from build123d import *

# Parameters (mm, degrees)
BOSS_EXTRUDE1_DEPTH     = 40
SKETCH2_W               = 10
SKETCH2_H               = 10
BOSS_EXTRUDE2_DEPTH     = 80
SKETCH3_R               = 1.5
CUT_EXTRUDE1_DEPTH      = 48.749345545
SKETCH4_R               = 1.5
BOSS_EXTRUDE3_DEPTH     = 10
CHAMFER1_SIZE           = 23.551326066
CHAMFER1_SIZE_2         = 12
CHAMFER2_SIZE           = 4
CHAMFER3_SIZE           = 4
CHAMFER4_SIZE           = 12
SKETCH7_R               = 1.5
CUT_EXTRUDE3_DEPTH      = 104.330973091
CUT_EXTRUDE2_DEPTH      = 103.553839519
CUT_EXTRUDE2_DEPTH_BACK = 2
CHAMFER5_SIZE           = 7
SKETCH8_R               = 5.15
CUT_EXTRUDE4_DEPTH      = 5.5
SKETCH9_R               = 2.75
CUT_EXTRUDE5_DEPTH      = 95.417371283
CHAMFER6_SIZE           = 2.5


# Some blends are built 0.0001 mm under size
with BuildPart() as part:
    # Sketch1 → Boss-Extrude1 (new, symmetric)
    with BuildSketch(Plane(origin=(0, 0, 0), x_dir=(0, 0, -1), z_dir=(1, 0, 0))):
        Polygon((0, 4), (0, 15), (-4, 15), (-4, -15), (0, -15), (0, -4), (1, -4), (1, 4), align=None)
    extrude(amount=BOSS_EXTRUDE1_DEPTH, both=True)

    # Sketch2 → Boss-Extrude2 (add)
    with BuildSketch(Plane.ZY.offset(40)):
        with Locations((9, -2)):
            Rectangle(SKETCH2_W, SKETCH2_H)
    extrude(amount=-BOSS_EXTRUDE2_DEPTH)

    # Sketch3 → Cut-Extrude1 (cut, through all)
    with BuildSketch(Plane.XZ.offset(7)):
        with Locations(Location((-28.7, 7.55, 0), (0, 0, 270))):
            Circle(SKETCH3_R)
        with Locations(Location((28.7, 7.55, 0), (0, 0, 270))):
            Circle(SKETCH3_R)
    extrude(amount=-CUT_EXTRUDE1_DEPTH, mode=Mode.SUBTRACT)

    # Sketch4 → Boss-Extrude3 (add)
    with BuildSketch(Plane.XZ.offset(7)):
        Polygon((-40, 14), (-29.75, 14), (-29.75, 72.7), (-25.75, 72.7), (-25.75, 84.7), (25.75, 84.7), (25.75, 72.7), (29.75, 72.7), (29.75, 14), (40, 14), (40, 92.7), (-40, 92.7), align=None)
        with Locations(Location((-28.7, 77.65, 0), (0, 0, 270))):
            Circle(SKETCH4_R, mode=Mode.SUBTRACT)
        with Locations(Location((28.7, 77.65, 0), (0, 0, 90))):
            Circle(SKETCH4_R, mode=Mode.SUBTRACT)
    extrude(amount=-BOSS_EXTRUDE3_DEPTH)

    # Chamfer1
    # the kernel refuses this chamfer: 23.551326066, 12 mm, written as the material it adds along each edge
    with BuildSketch(Plane(origin=(-40, 3, 4), x_dir=(0, -0.017531984409911095, 0.9998463029499337), z_dir=(1, 0, 0))) as chamfer1_piece_1_section:
        Polygon((CHAMFER1_SIZE * 0.999846302953, -CHAMFER1_SIZE * 0.01753198441), (-CHAMFER1_SIZE_2 * 0.0175319844099, -CHAMFER1_SIZE_2 * 0.99984630295), (0, 0), align=None)
    chamfer1_piece_1 = extrude(amount=80, mode=Mode.PRIVATE)
    chamfer1_piece_1 = split(chamfer1_piece_1, bisect_by=Plane(origin=(-34.875, 4.887878827, 14), z_dir=(0, 0, 1)), keep=Keep.TOP, mode=Mode.PRIVATE)
    chamfer1_piece_1 = split(chamfer1_piece_1, bisect_by=Plane(origin=(-29.75, 4.887878827, 19.058840597), z_dir=(-1, 0, 0)), keep=Keep.TOP, mode=Mode.PRIVATE)
    add(chamfer1_piece_1)
    with BuildSketch(Plane(origin=(-40, 3, 4), x_dir=(0, -0.017531984409911095, 0.9998463029499337), z_dir=(1, 0, 0))) as chamfer1_piece_2_section:
        Polygon((CHAMFER1_SIZE * 0.999846302953, -CHAMFER1_SIZE * 0.01753198441), (-CHAMFER1_SIZE_2 * 0.0175319844099, -CHAMFER1_SIZE_2 * 0.99984630295), (0, 0), align=None)
    chamfer1_piece_2 = extrude(amount=80, mode=Mode.PRIVATE)
    chamfer1_piece_2 = split(chamfer1_piece_2, bisect_by=Plane(origin=(-34.907327213, 7.791187199, 14), z_dir=(0, 0, -1)), keep=Keep.TOP, mode=Mode.PRIVATE)
    chamfer1_piece_2 = split(chamfer1_piece_2, bisect_by=Plane(origin=(-29.75, 7.791187199, 8.24071688), z_dir=(-1, 0, 0)), keep=Keep.TOP, mode=Mode.PRIVATE)
    chamfer1_piece_2 = chamfer1_piece_2 - Plane(origin=(-28.7, 7.791187199, 7.55), x_dir=(0, 0, -1), z_dir=(0, -1, 0)) * Cylinder(1.5, 255, mode=Mode.PRIVATE)
    chamfer1_piece_2 = split(chamfer1_piece_2, bisect_by=Plane(origin=(-34.907327213, 15, 8.24071688), z_dir=(0, -1, 0)), keep=Keep.TOP, mode=Mode.PRIVATE)
    add(chamfer1_piece_2)
    with BuildSketch(Plane(origin=(-40, 3, 4), x_dir=(0, -0.017531984409911095, 0.9998463029499337), z_dir=(1, 0, 0))) as chamfer1_piece_3_section:
        Polygon((CHAMFER1_SIZE * 0.999846302953, -CHAMFER1_SIZE * 0.01753198441), (-CHAMFER1_SIZE_2 * 0.0175319844099, -CHAMFER1_SIZE_2 * 0.99984630295), (0, 0), align=None)
    chamfer1_piece_3 = extrude(amount=80, mode=Mode.PRIVATE)
    chamfer1_piece_3 = split(chamfer1_piece_3, bisect_by=Plane(origin=(3.218e-06, 7.789653484, 14), z_dir=(0, 0, -1)), keep=Keep.TOP, mode=Mode.PRIVATE)
    chamfer1_piece_3 = split(chamfer1_piece_3, bisect_by=Plane(origin=(-29.75, 7.789653484, 8.251914963), z_dir=(1, 0, 0)), keep=Keep.TOP, mode=Mode.PRIVATE)
    chamfer1_piece_3 = split(chamfer1_piece_3, bisect_by=Plane(origin=(29.75, 7.789653484, 8.251914963), z_dir=(-1, 0, 0)), keep=Keep.TOP, mode=Mode.PRIVATE)
    chamfer1_piece_3 = chamfer1_piece_3 - Plane(origin=(28.7, 7.789653484, 7.55), x_dir=(0, 0, -1), z_dir=(0, -1, 0)) * Cylinder(1.5, 255, mode=Mode.PRIVATE)
    chamfer1_piece_3 = chamfer1_piece_3 - Plane(origin=(-28.7, 7.789653484, 7.55), x_dir=(0, 0, -1), z_dir=(0, -1, 0)) * Cylinder(1.5, 255, mode=Mode.PRIVATE)
    chamfer1_piece_3 = split(chamfer1_piece_3, bisect_by=Plane(origin=(3.218e-06, 15, 8.251914963), z_dir=(0, -1, 0)), keep=Keep.TOP, mode=Mode.PRIVATE)
    add(chamfer1_piece_3)
    with BuildSketch(Plane(origin=(-40, 3, 4), x_dir=(0, -0.017531984409911095, 0.9998463029499337), z_dir=(1, 0, 0))) as chamfer1_piece_4_section:
        Polygon((CHAMFER1_SIZE * 0.999846302953, -CHAMFER1_SIZE * 0.01753198441), (-CHAMFER1_SIZE_2 * 0.0175319844099, -CHAMFER1_SIZE_2 * 0.99984630295), (0, 0), align=None)
    chamfer1_piece_4 = extrude(amount=80, mode=Mode.PRIVATE)
    chamfer1_piece_4 = split(chamfer1_piece_4, bisect_by=Plane(origin=(34.875, 4.887878827, 14), z_dir=(0, 0, 1)), keep=Keep.TOP, mode=Mode.PRIVATE)
    chamfer1_piece_4 = split(chamfer1_piece_4, bisect_by=Plane(origin=(29.75, 4.887878827, 19.058840597), z_dir=(1, 0, 0)), keep=Keep.TOP, mode=Mode.PRIVATE)
    add(chamfer1_piece_4)
    with BuildSketch(Plane(origin=(-40, 3, 4), x_dir=(0, -0.017531984409911095, 0.9998463029499337), z_dir=(1, 0, 0))) as chamfer1_piece_5_section:
        Polygon((CHAMFER1_SIZE * 0.999846302953, -CHAMFER1_SIZE * 0.01753198441), (-CHAMFER1_SIZE_2 * 0.0175319844099, -CHAMFER1_SIZE_2 * 0.99984630295), (0, 0), align=None)
    chamfer1_piece_5 = extrude(amount=80, mode=Mode.PRIVATE)
    chamfer1_piece_5 = split(chamfer1_piece_5, bisect_by=Plane(origin=(34.907327332, 7.791187313, 14), z_dir=(0, 0, -1)), keep=Keep.TOP, mode=Mode.PRIVATE)
    chamfer1_piece_5 = split(chamfer1_piece_5, bisect_by=Plane(origin=(29.75, 7.791187313, 8.240716948), z_dir=(1, 0, 0)), keep=Keep.TOP, mode=Mode.PRIVATE)
    chamfer1_piece_5 = chamfer1_piece_5 - Plane(origin=(28.7, 7.791187313, 7.55), x_dir=(0, 0, -1), z_dir=(0, -1, 0)) * Cylinder(1.5, 255, mode=Mode.PRIVATE)
    chamfer1_piece_5 = split(chamfer1_piece_5, bisect_by=Plane(origin=(34.907327332, 15, 8.240716948), z_dir=(0, -1, 0)), keep=Keep.TOP, mode=Mode.PRIVATE)
    add(chamfer1_piece_5)

    # Chamfer2
    chamfer2_edges = [part.edges().sort_by_distance(p)[0] for p in [
        (-29.75, -2, 72.7),
        (29.75, -2, 72.7),
    ]]
    chamfer(chamfer2_edges, length=CHAMFER2_SIZE - 0.0001)  # a hair under: the kernel refuses the full size

    # Chamfer3
    chamfer3_edges = [part.edges().sort_by_distance(p)[0] for p in [
        (0, 3, 92.7),
    ]]
    chamfer(chamfer3_edges, length=CHAMFER3_SIZE)

    # Chamfer4
    chamfer4_edges = [part.edges().sort_by_distance(p)[0] for p in [
        (-25.75, -2, 84.7),
        (25.75, -2, 84.7),
        (29.75, 1.452372753, 14),
        (-29.75, 1.452372753, 14),
    ]]
    chamfer(chamfer4_edges, length=CHAMFER4_SIZE - 0.0001)  # a hair under: the kernel refuses the full size

    # Sketch7 → Cut-Extrude3 (cut, through all)
    with BuildSketch(Plane.XZ.offset(7)):
        with Locations(Location((-33, 85.7, 0), (0, 0, 270))):
            Circle(SKETCH7_R)
        with Locations(Location((33, 85.7, 0), (0, 0, 270))):
            Circle(SKETCH7_R)
    extrude(amount=-CUT_EXTRUDE3_DEPTH, mode=Mode.SUBTRACT)

    # Sketch5 → Cut-Extrude2 (cut, two sides: drawn at the far end of the back side and taken through both)
    with BuildSketch(Plane(origin=(0, 3, 0), x_dir=(1, 0, 0), z_dir=(0, 1, 0)).offset(-CUT_EXTRUDE2_DEPTH_BACK)):
        Polygon((32.164101615, -77.65), (30.432050808, -80.65), (26.967949192, -80.65), (25.235898385, -77.65), (26.967949192, -74.65), (30.432050808, -74.65), align=None)
        Polygon((-26.967949192, -74.65), (-30.432050808, -74.65), (-32.164101615, -77.65), (-30.432050808, -80.65), (-26.967949192, -80.65), (-25.235898385, -77.65), align=None)
        Polygon((-25.235898385, -7.55), (-26.967949192, -10.55), (-30.432050808, -10.55), (-32.164101615, -7.55), (-30.432050808, -4.55), (-26.967949192, -4.55), align=None)
        Polygon((26.967949192, -10.55), (30.432050808, -10.55), (32.164101615, -7.55), (30.432050808, -4.55), (26.967949192, -4.55), (25.235898385, -7.55), align=None)
    extrude(amount=CUT_EXTRUDE2_DEPTH + CUT_EXTRUDE2_DEPTH_BACK, mode=Mode.SUBTRACT)

    # Chamfer5
    chamfer5_edges = [part.edges().sort_by_distance(p)[0] for p in [
        (-40, -4, 92.7),
        (40, -4, 92.7),
    ]]
    chamfer(chamfer5_edges, length=CHAMFER5_SIZE)

    # Sketch8 → Cut-Extrude4 (cut)
    with BuildSketch(Plane.XY.offset(14)):
        Circle(SKETCH8_R)
    extrude(amount=-CUT_EXTRUDE4_DEPTH, mode=Mode.SUBTRACT)

    # Sketch9 → Cut-Extrude5 (cut, through all)
    with BuildSketch(Plane.XY.offset(8.5)):
        Circle(SKETCH9_R)
    extrude(amount=-CUT_EXTRUDE5_DEPTH, mode=Mode.SUBTRACT)

    # Chamfer6
    # the kernel refuses this chamfer: 2.5 mm, written as the material it takes off along each edge
    with BuildSketch(Plane(origin=(0, 0, 8.5), x_dir=(1, 0, 0), z_dir=(0, -1, 0))) as chamfer6_piece_1_section:
        Polygon((2.75, -CHAMFER6_SIZE), (2.75 + CHAMFER6_SIZE, 0), (2.75, 0), align=None)
    chamfer6_piece_1 = revolve(axis=Axis((0, 0, 8.5), (0, 0, 1)), mode=Mode.PRIVATE)
    chamfer6_piece_1 = chamfer6_piece_1 & Plane(origin=(0, 0, 7.19466401), x_dir=(1, 0, 0), z_dir=(0, 0, 1)) * Cylinder(5.15, 21, mode=Mode.PRIVATE)
    add(chamfer6_piece_1, mode=Mode.SUBTRACT)


solid = part.part
Input: part model. Units: mm. Frame: model coordinates. A direction names the side the tool comes from. Give positions to 0.01 mm unless a question says otherwise; leave off trailing zeros. Write each loop counter-clockwise with the first axis right and the second up, starting at its lowest first coordinate (ties: lowest second). Pieces come first, ordered by that corner, then holes.
Q1. Material intervals for probe 1 along X at (y, z) = (-5, 85.7); probe 2 along X at (y, z) = (-5, 7.55); probe 3 along Z at (x, y) = (-8.5, -9.5), sorted ascending.
Q2. First-contact query: P1, Ø1.7, axis at x = -29.5, y = 10.5, coming from the +Z side; P2, Ø5, axis at x = 28, z = 8.5, coming from the +Y side; P3, Ø6.5, axis at x = 0.5, y = -12.5, coming from the +Z side. Flat tips, straight axial feed; report the tip coordinate or a pass-through.
Q3. Set-up query: faces 4 (the face through (-27.78, -2.07, 70.67)), 5 (the face through (31.286, 7.01, 9.071)). Return all of +Z, -Z, +X, -X, +Y, -Y with unobstructed straight access to the full face (end or side cutting, diameter ignored); none if empty.
Q4. Section B-B, the plane z = 67. Output: boundary loops of the cut face in (x, y), plus the area to 3 significant figures.
Q5. Section A-A, the plane x = -12. Output: boundary loops of the cut face in (y, z), plus the area to 3 significant figures.
Q6. Pull-direction query (X, two-part tool) for faces 1 (the face through (36.5, -2.1, 89.2)), 2 (the face through (1, -11, 4)), 3 (the face through (28, 1, 76)); classes: pulls with the +X half, pulls with the -X half, needs draft (parallel to the pull), parting line crosses it, or undercut.
Q7. Section C-C, the plane x = 0. Output: boundary loops of the cut face in (y, z), plus the area to 3 significant figures.
Q8. Section D-D, the plane y = 8.5. Output: boundary loops of the cut face in (x, z).
Filled in:
1. probe 1: x = -40 to -34.5, -31.5 to 31.5, 34.5 to 40
1. probe 2: x = -40 to -30.2, -27.2 to 27.2, 30.2 to 40
1. probe 3: z = 0 to 4
2. P1: stops at z = 14.5
2. P2: stops at y = 12.93
2. P3: stops at z = 4
3. face 4: +Y, -Y
3. face 5: +Y
4. outline: (-40, -7) - (-29.75, -7) - (-29.75, 3) - (-40, 3) - close; (29.75, -7) - (40, -7) - (40, 3) - (29.75, 3) - close
4. area: 205 mm2
5. outline: (-15, 0) - (-4, 0) - (-4, -1) - (4, -1) - (4, 0) - (15, 0) - (15, 4) - (9.9, 14) - (-7, 14) - (-7, 4) - (-15, 4) - close; (-7, 84.7) - (3, 84.7) - (3, 88.7) - (-1, 92.7) - (-7, 92.7) - close
5. area: 395 mm2
6. face 1: pulls with the +X half
6. face 2: needs draft
6. face 3: undercut
7. outline: (-15, 0) - (-4, 0) - (-4, -1) - (-2.75, -1) - (-2.75, 6) - (-5.15, 8.4) - (-5.15, 14) - (-7, 14) - (-7, 4) - (-15, 4) - close; (-7, 84.7) - (3, 84.7) - (3, 88.7) - (-1, 92.7) - (-7, 92.7) - close; (2.75, -1) - (4, -1) - (4, 0) - (15, 0) - (15, 4) - (9.9, 14) - (5.15, 14) - (5.15, 8.4) - (2.75, 6) - close
7. area: 279 mm2
8. outline: (-40, 0) - (40, 0) - (40, 16.76) - (20.51, 16.76) - (17.75, 14) - (-17.75, 14) - (-20.51, 16.76) - (-40, 16.76) - close; hole (-32.16, 7.55) - (-30.43, 4.55) - (-26.97, 4.55) - (-25.24, 7.55) - (-26.97, 10.55) - (-30.43, 10.55) - close; hole (25.24, 7.55) - (26.97, 4.55) - (30.43, 4.55) - (32.16, 7.55) - (30.43, 10.55) - (26.97, 10.55) - close
